Check sheet for the drawn part. Datum: minimum x, y, z corner. Units: mm. Coordinates: 2 decimals unless noted, no trailing zeros. Order: outer loops, then holes, each group sorted by start corner. A loop starts at its lowest first (then second) coordinate and runs counter-clockwise, first axis right, second up. Notation, with made-up numbers: (-13, -24) - (36, -24) arc R11 cw to (36, -13) - close; hole circle Ø10 at (0.5, 86.25). An arc over 180 degrees is marked (long way). Return JSON: item names as keys, results as strings. Group by question number.
Item 1: Section check C-C on x = 18.5. Enter the section's corners in (y, z), then the cut area to 3 significant figures.
Item 2: Scan lines: probe 1 along X at (y, z) = (24, 0.8); probe 2 along Y at (x, z) = (66.9, 1); probe 3 along Y at (x, z) = (78.5, 2). Record each from-to range of solid material in increasing order.
Item 3: Gauge pin test, flat end, axial feed: pin 1 (3 mm diameter, centred on x = 30.1, y = 22.5, fed in from +Z). Record the tip position at first contact, or that the pin passes through.
Item 4: Section check B-B on z = 1.3. Enter the section's corners in (x, y), then the cut area to 3 significant figures.
Item 5: Section check A-A on y = 22.5. Enter the section's corners in (x, z), then the cut area to 3 significant figures.
Item 6: Section check D-D on x = 66.9. Enter the section's corners in (y, z).
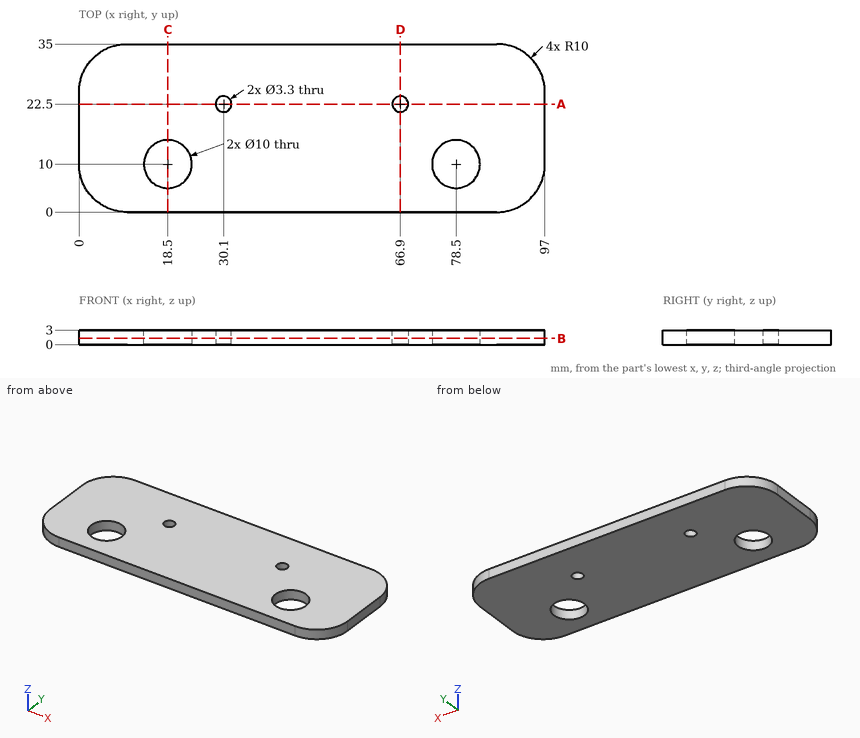
Computed:
{
 "1": {"outline": "(0, 0) - (5, 0) - (5, 3) - (0, 3) - close; (15, 0) - (35, 0) - (35, 3) - (15, 3) - close", "area": "75.0 mm²"},
 "2": {"probe 1": "x = 0 to 29.41, 30.79 to 66.21, 67.59 to 97", "probe 2": "y = 0 to 20.85, 24.15 to 35", "probe 3": "y = 0 to 5, 15 to 35"},
 "3": {"pin 1": "passes through"},
 "4": {"outline": "(0, 10) arc R10 ccw to (10, 0) - (87, 0) arc R10 ccw to (97, 10) - (97, 25) arc R10 ccw to (87, 35) - (10, 35) arc R10 ccw to (0, 25) - close; hole circle Ø10 at (18.5, 10); hole circle Ø3.3 at (30.1, 22.5); hole circle Ø3.3 at (66.9, 22.5); hole circle Ø10 at (78.5, 10)", "area": "3,130 mm²"},
 "5": {"outline": "(0, 0) - (28.45, 0) - (28.45, 3) - (0, 3) - close; (31.75, 0) - (65.25, 0) - (65.25, 3) - (31.75, 3) - close; (68.55, 0) - (97, 0) - (97, 3) - (68.55, 3) - close", "area": "271 mm²"},
 "6": {"outline": "(0, 0) - (20.85, 0) - (20.85, 3) - (0, 3) - close; (24.15, 0) - (35, 0) - (35, 3) - (24.15, 3) - close"}
}
